Source: CAD feature listing. Evaluate the final solid. Frame: model axes, mm. A direction names the side the tool comes from. Round coordinates to 2 decimals unless told otherwise and drop trailing zeros. Loops run counter-clockwise (first coordinate to the right, second up) from the corner with the lowest first, then second, coordinate; pieces in that order, holes last. Notation, with made-up numbers: (-1.75, 42) - (2.25, 42) arc R22 ccw to (2.25, 69) - close; hole circle Ø8 at (-39, 2.25). An arc over 180 degrees is marked (long way). One line per question, with ' | ' between items.
Autodesk Fusion 360 part; units mm, degrees
sketch "Sketch1" plane through (0, 0, 0) normal (0, 1, 0) x (1, 0, 0)
  circle A0 centre (0, 0) radius 5
  circle A1 centre (0, 0) radius 11
  circle A2 centre (0, 0) radius 4
  circle A3 centre (8, 0) radius 2
  circle A4 centre (0, 8) radius 2
  circle A5 centre (-8, 0) radius 2
  circle A6 centre (0, -8) radius 2
  dimension "d1" = 10
  dimension "d8" = 22
  dimension "d11" = 8
  dimension "d15" = 4
  dimension "d17" = 4
  dimension "d18" = 4
  dimension "d19" = 4
sketch "Sketch2" plane through (0, 0, 0) normal (0, 1, 0) x (1, 0, 0)
  line L0 (-25, 25) -> (25, 25)
  line L1 (25, 25) -> (25, -25)
  line L2 (25, -25) -> (-25, -25)
  line L3 (-25, -25) -> (-25, 25)
extrude "Extrude1" add sketch "Sketch1" along normal blind 3 contours A0 | A1 in component "Component"
extrude "Extrude2" add sketch "Sketch1" along normal blind 13 and the other way blind 2 contours A0 in component "Component"
chamfer "Chamfer1" distance 0.1 angle 45 16 edges at (-9.8647, 3, -0.7232) (-3.7293, 13, -1.4465) (-4.6616, 3, -1.8081) (6.1353, 3, -0.7232) (-1.8647, 3, -8.7232) (-1.8647, 3, 7.2768) (-4.6616, -2, -1.8081) (-10.2556, 0, 3.9778) (-4.6616, 13, 1.8081) (6.1353, 0, -0.7232) (-9.8647, 0, -0.7232) (-10.2556, 3, 3.9778) (-1.8647, 0, 7.2768) (-3.7293, -2, 1.4465) (-4.6616, 0, 1.8081) (-1.8647, 0, -8.7232) in component "Component"
component "Component" placed x (1, 0, 0) y (0, 1, 0) z (0, 0, 1) at (0, 0, 0)
1. Access query for faces 5 (the flat face through (5, 3, 2)), 6 (the cylindrical face through (0, 1, 10)). Directions: +Z, -Z, +X, -X, +Y, -Y. A direction counts if a zero-diameter tool reaches every point of the face in a straight line with its end or side. Return the directions, or none.
Worked out:
face 5: +Y | face 6: +Y, -Y
2. Material intervals for probe 1 along Z at (x, y) = (0, 2.25); probe 2 along X at (y, z) = (9, 0), sorted ascending.
Worked out:
probe 1: z = -11 to -10, -6 to -4, 4 to 6, 10 to 11 | probe 2: x = -5 to -4, 4 to 5
3. Section query C-C, the plane y = -1. Return loops of the section in (x, z).
Worked out:
outline: circle Ø10 at (0, 0); hole circle Ø8 at (0, 0)
4. Contact query for flat-ended pins moving along their axis: P1, Ø1, axis at y = 2.5, z = 7.5, coming from the +X side; P2, Ø8, axis at y = 2.5, z = 5.5, coming from the +X side; P3, Ø2, axis at x = -1, y = 10.5, coming from the +Z side. Output: stop coordinate, or through.
Worked out:
P1: stops at x = 8.49 | P2: stops at x = 10.9 | P3: stops at z = 5
5. Section query A-A, the plane x = 0. Give the number of separate pieces and of enclosed holes in the cut face, plus the area to 3 significant figures.
Worked out:
separate pieces: 4 | enclosed holes: 0 | area: 41.9 mm2
6. Mould query, pull axis X, two halves, no side actions, for faces 1 (the cylindrical face through (6, 1, 0)), 2 (the cylindrical face through (0, 1, -6)), 3 (the cylindrical face through (-2.38, 1.48, -10.74)), 4 (the flat face through (2, 13, 4)). Classes: released by +X, released by -X, zero draft, split by the parting line, or undercut.
Worked out:
face 1: undercut | face 2: undercut | face 3: split by the parting line | face 4: zero draft
